The listing builds one solid part. Answer for the finished solid, in the listing's coordinates (mm). A direction names the side the tool comes from. Coordinates: 2 decimals unless noted, no trailing zeros. Order: outer loops, then holes, each group sorted by start corner. A loop starts at its lowest first (then second) coordinate and runs counter-clockwise, first axis right, second up.
```python
from build123d import *

# Parameters (mm, degrees)
F0_R     = 34.44374921
F1_DEPTH = 25.4
F2_SIZE  = 5.08
F3_SIZE  = 5.08
F4_DEPTH = 25.4
F5_SIZE  = 5.08
F6_DEPTH = 25.4
F7_SIZE  = 5.08
F8_SIZE  = 5.08


# Not quite as in the source:
# - two fillets or chamfers of one size are made in one step


with BuildPart() as f1:
    # F0 (on Top) → F1 (new body)
    with BuildSketch(Plane.XY):
        with Locations((-39.9288013577, 17.5260007381)):
            Circle(F0_R)
    extrude(amount=F1_DEPTH)

    # F2
    f2_edges = [f1.edges().sort_by_distance(p)[0] for p in [
        (-74.372551, 17.526001, 25.4),
    ]]
    chamfer(f2_edges, length=F2_SIZE)

    # F3
    f3_edges = [f1.edges().sort_by_distance(p)[0] for p in [
        (-74.372551, 17.526001, 20.32),
    ]]
    chamfer(f3_edges, length=F3_SIZE)

    # F4 (add): a face of the model
    f4_faces = [f1.faces().sort_by_distance(p)[0] for p in [
        (-39.9288013577, 17.5260007381, 25.4),
    ]]
    extrude(f4_faces, amount=F4_DEPTH)

    # F5
    f5_edges = [f1.edges().sort_by_distance(p)[0] for p in [
        (-69.292551, 17.526001, 50.8),
    ]]
    chamfer(f5_edges, length=F5_SIZE)

    # F6 (add): a face of the model
    f6_faces = [f1.faces().sort_by_distance(p)[0] for p in [
        (-39.9288013577, 17.5260007381, 50.8),
    ]]
    extrude(f6_faces, amount=F6_DEPTH)

    # F7
    f7_edges = [f1.edges().sort_by_distance(p)[0] for p in [
        (-69.292551, 17.526001, 45.72),
        (-64.212551, 17.526001, 76.2),
    ]]
    chamfer(f7_edges, length=F7_SIZE)

    # F8
    f8_edges = [f1.edges().sort_by_distance(p)[0] for p in [
        (-64.212551, 17.526001, 71.12),
    ]]
    chamfer(f8_edges, length=F8_SIZE)


solid = f1.part
```
(1) Consider line 1 (Y direction, x = -54, z = 31.5); line 2 (X direction, y = 16.5, z = 64); line 3 (X direction, y = 34.5, z = 43). Determine where each line is inside the solid, lowest interval first.
(2) Each of these flat-tipped pins is pushed along its axis until it touches: pin 1 Ø1.5 at (x, z) = (-50.5, 64) entering from +Y; pin 2 Ø8 at (x, z) = (-46.5, 63.5) entering from -Y; pin 3 Ø4 at (x, z) = (-62.5, 36.5) entering from -Y; pin 4 Ø1.5 at (x, z) = (-65, 65) entering from +Y. Where does it stop, or does it pass through?
(3) Find section B-B (z = 57.5). Write down the section's boundary in (x, y).
(4) For faces 1 (the face through (-59.2, 2.75, 58.31)), 2 (the face through (-40, 18, 0)), determine the directions among +Z, -Z, +X, -X, +Y, -Y from which every point of the face is accessible in a straight line to the end or side of a thin tool.
(5) Find section A-A (z = 37). Write down the section's boundary in (x, y), and give its area (3 significant figures).
Findings below:
1. line 1: y = -8.25 to 43.3
1. line 2: x = -64.19 to -15.67
1. line 3: x = -62.68 to -17.18
2. pin 1: stops at y = 39.74
2. pin 2: stops at y = -6.62
2. pin 3: stops at y = -3.43
2. pin 4: passes through
3. outline: circle Ø48.57 at (-39.93, 17.53)
4. face 1: +Z
4. face 2: -Z, +X, -X, +Y, -Y
5. outline: circle Ø58.73 at (-39.93, 17.53)
5. area: 2,710 mm2
